Verification items for this drawing (mm, ordinates from the low corner). Give positions to 0.01 mm unless a question says otherwise; leave off trailing zeros. Order: outer loops, then holes, each group sorted by start corner. A loop starts at its lowest first (then second) coordinate and runs counter-clockwise, first axis right, second up. Notation, with made-up numbers: M 57.5,-36 L 85.5,-36 A19 ccw 85.5,-5 Z; hole C -20,-18 d8. An arc over 180 degrees is marked long. Return JSON: item names as keys, results as strings. Group by question number.
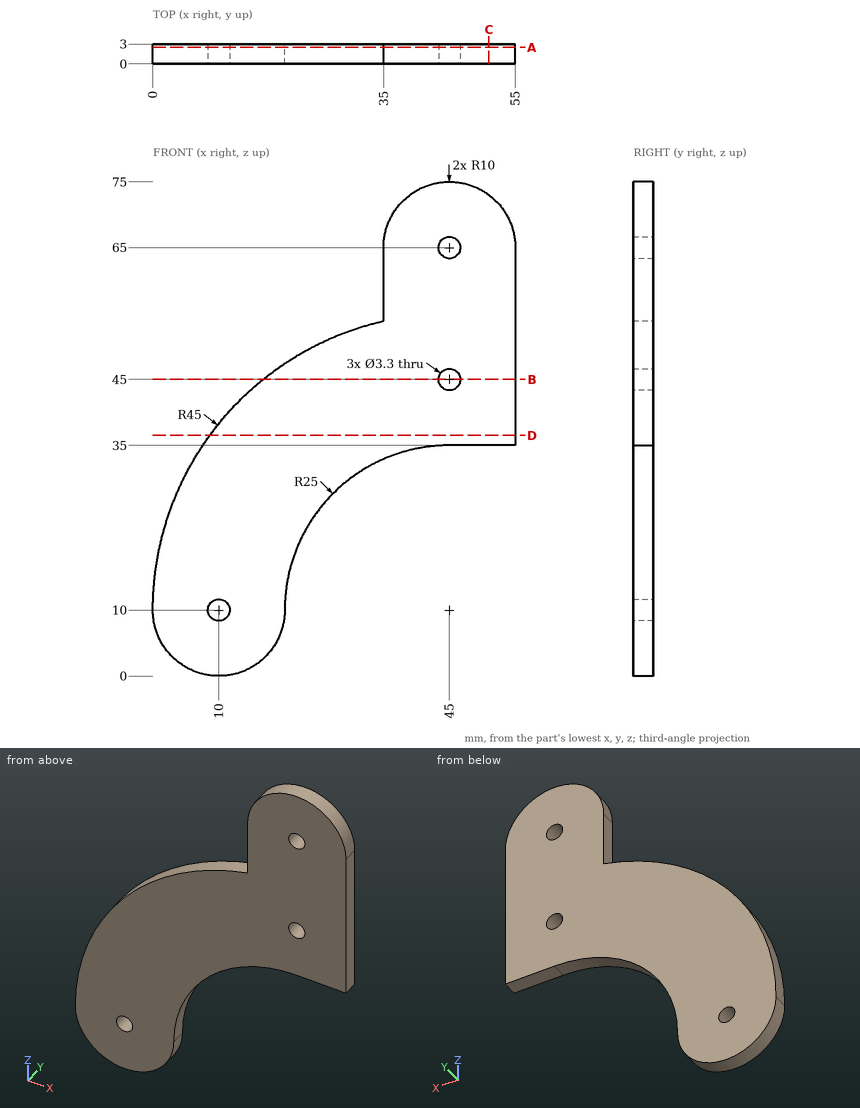
1) Depth check by flat-ended pin: P1, Ø12, axis at x = 16.5, z = 17, coming from the -Y side; P2, Ø2.5, axis at x = 10, z = 10, coming from the -Y side; P3, Ø1.5, axis at x = 20, y = 0.5, coming from the +Z side; P4, Ø1, axis at y = 1.5, z = 29.5, coming from the -X side. Enter the tip coordinate at first touch or a pass-through.
2) Material ranges on line 1 along X through (y, z) = (0.6, 65); line 2 along X through (y, z) = (0.95, 10); line 3 along Z through (x, y) = (17.5, 0.7), recorded low to high.
3) Sectioned sample at D-D on z = 36.5. Record the boundary of the cut face in (x, y), then the cut area to 3 significant figures.
4) Sectioned sample at B-B on z = 45. Record the boundary of the cut face in (x, y), then the cut area to 3 significant figures.
5) Sectioned sample at A-A on y = 2.5. Record the boundary of the cut face in (x, z).
6) Sectioned sample at C-C on x = 51. Record the boundary of the cut face in (y, z).
Reply:
{
 "1": {"P1": "y = 0", "P2": "through", "P3": "z = 47.91", "P4": "x = 4.21"},
 "2": {"line 1": "35 to 43.35, 46.65 to 55", "line 2": "0 to 8.35, 11.65 to 20", "line 3": "3.39 to 45.62"},
 "3": {"outline": "M 8.63,0 L 55,0 L 55,3 L 8.63,3 Z", "area": "139 mm^2"},
 "4": {"outline": "M 16.72,0 L 43.35,0 L 43.35,3 L 16.72,3 Z; M 46.65,0 L 55,0 L 55,3 L 46.65,3 Z", "area": "105 mm^2"},
 "5": {"outline": "M 0,10 A10 ccw 20,10 A25 cw 45,35 L 55,35 L 55,65 A10 ccw 35,65 L 35,53.87 A45 ccw Z; hole C 10,10 d3.3; hole C 45,45 d3.3; hole C 45,65 d3.3"},
 "6": {"outline": "M 0,35 L 3,35 L 3,73 L 0,73 Z"}
}
